from build123d import *

# Parameters (mm, degrees)
F0_W     = 70.5
F0_H     = 10
F1_DEPTH = 6
F3_DEPTH = 0.508
F4_W     = 2
F4_H     = 8
F5_DEPTH = 15


with BuildPart() as f1:
    # F0 (on Front) → F1 (new body)
    with BuildSketch(Plane.XZ):
        with Locations((22.643538, 41.13415)):
            Rectangle(F0_W, F0_H)
    extrude(amount=F1_DEPTH)

    # F2 (on face) → F3 (cut)
    with BuildSketch(Plane.XZ.offset(6)):
        Polygon((-5.727013, 46.13415), (-12.606462, 36.13415), (-10.066462, 36.13415), (-3.187013, 46.13415), align=None)
        Polygon((4.432987, 46.13415), (1.892987, 46.13415), (-4.986462, 36.13415), (-2.446462, 36.13415), align=None)
        Polygon((12.052987, 46.13415), (9.512987, 46.13415), (2.633538, 36.13415), (5.173538, 36.13415), align=None)
        Polygon((19.672987, 46.13415), (17.132987, 46.13415), (10.253538, 36.13415), (12.793538, 36.13415), align=None)
        Polygon((27.292987, 46.13415), (24.752987, 46.13415), (17.873538, 36.13415), (20.413538, 36.13415), align=None)
        Polygon((34.912987, 46.13415), (32.372987, 46.13415), (25.493538, 36.13415), (28.033538, 36.13415), align=None)
        Polygon((42.532987, 46.13415), (39.992987, 46.13415), (33.113538, 36.13415), (35.653538, 36.13415), align=None)
        Polygon((50.152987, 46.13415), (47.612987, 46.13415), (40.733538, 36.13415), (43.273538, 36.13415), align=None)
        Polygon((57.772987, 46.13415), (55.232987, 46.13415), (48.353538, 36.13415), (50.893538, 36.13415), align=None)
    extrude(amount=-F3_DEPTH, mode=Mode.SUBTRACT)

    # F4 (on face) → F5 (cut)
    with BuildSketch(Plane(origin=(-12.606462, 0, 0), x_dir=(0, -1, 0), z_dir=(-1, 0, 0))):
        with Locations((2.5, 41.13415)):
            Rectangle(F4_W, F4_H)
    extrude(amount=-F5_DEPTH, mode=Mode.SUBTRACT)


solid = f1.part
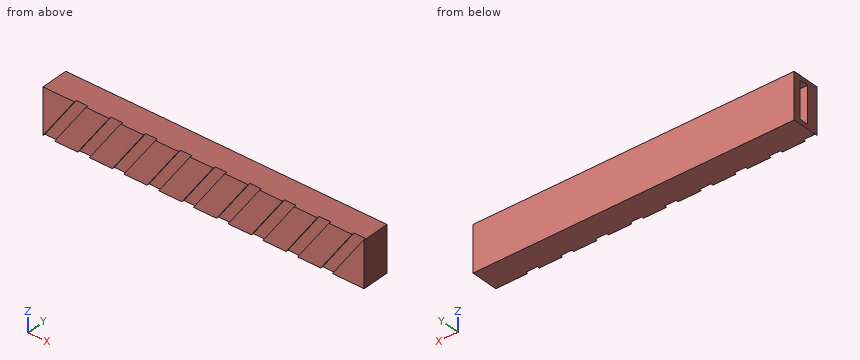
The model under review builds one solid part; all positions refer to its coordinate system, in mm. Give positions to 0.01 mm unless a question says otherwise; leave off trailing zeros. Order: outer loops, then holes, each group sorted by start corner. A loop starts at its lowest first (then second) coordinate and runs counter-clockwise, first axis right, second up. Notation, with made-up numbers: M 57.25,10.25 L 79.25,10.25 A17 ccw 79.25,21.25 Z; hole C 65,0.5 d8. An arc over 180 degrees is marked long. Answer in a Markdown table with one row per item. Add a question column.
1. Add section B-B on x = 26.5. State the section outline as (y, z) points, plus the area to 3 significant figures.
2. Add section A-A on x = 46. State the section outline as (y, z) points.
3. To check wall thickness, follow line 1 along Y through (x, z) = (-2, 37.5); line 2 along Y through (x, z) = (-8, 39); line 3 along X through (y, z) = (-2.6, 43.5). State the ranges of each line that lie inside material, in increasing order.
The answers:
| question | item | result |
|---|---|---|
| 1 | outline | M -6,37.6 L -5.49,37.6 L -5.49,36.13 L 0,36.13 L 0,46.13 L -5.49,46.13 L -5.49,44.98 L -6,44.98 Z |
| 1 | area | 58.7 mm2 |
| 2 | outline | M -6,36.13 L 0,36.13 L 0,46.13 L -6,46.13 L -6,43.79 L -5.49,43.79 L -5.49,40.1 L -6,40.1 Z |
| 3 | line 1 | -5.49 to -3.5, -1.5 to 0 |
| 3 | line 2 | -6 to -3.5, -1.5 to 0 |
| 3 | line 3 | 2.39 to 57.89 |
